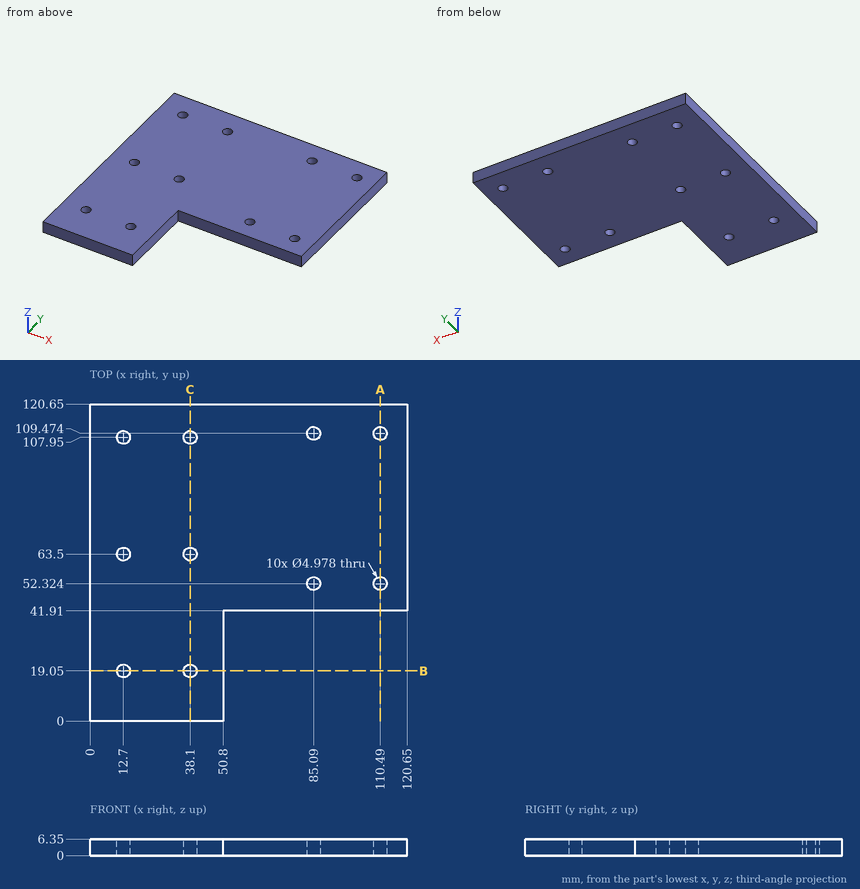
Input: dimensioned drawing with shaded views. Units: mm. Origin: part minimum x, y, z. Give positions to 0.01 mm unless a question says otherwise; leave off trailing zeros. Order: outer loops, then holes, each group sorted by start corner. A loop starts at its lowest first (then second) coordinate and runs counter-clockwise, first axis right, second up. Notation, with made-up numbers: (63, 17.25) -> (72, 17.25) arc R20 ccw to (72, 47.25) -> close; hole circle Ø11 at (61, 54). An arc over 180 degrees is marked (long way). Use a Markdown table: item, result.
1) Section query B-B, the plane y = 19.05. Return the cut outline in (x, z).
Answer list:
| item | result |
|---|---|
| outline | (0, 0) -> (10.21, 0) -> (10.21, 6.35) -> (0, 6.35) -> close; (15.19, 0) -> (35.61, 0) -> (35.61, 6.35) -> (15.19, 6.35) -> close; (40.59, 0) -> (50.8, 0) -> (50.8, 6.35) -> (40.59, 6.35) -> close |
2) Section query C-C, the plane x = 38.1. Return the cut outline in (y, z).
Answer list:
| item | result |
|---|---|
| outline | (0, 0) -> (16.56, 0) -> (16.56, 6.35) -> (0, 6.35) -> close; (21.54, 0) -> (61.01, 0) -> (61.01, 6.35) -> (21.54, 6.35) -> close; (65.99, 0) -> (105.46, 0) -> (105.46, 6.35) -> (65.99, 6.35) -> close; (110.44, 0) -> (120.65, 0) -> (120.65, 6.35) -> (110.44, 6.35) -> close |
3) Section query A-A, the plane x = 110.49. Count the separate pieces of the cut face and the enclosed holes in it, then the cut area to 3 significant figures.
Answer list:
| item | result |
|---|---|
| separate pieces | 3 |
| enclosed holes | 0 |
| area | 437 mm² |
4) Ray query, line 1 along Y through (x, z) = (12.7, 2.25); line 2 along Y through (x, z) = (59.5, 1.75); line 3 along Y through (x, z) = (40, 2.75). Return the intervals inside material, ascending. Write a range as [from, to].
Answer list:
| item | result |
|---|---|
| line 1 | [0, 16.56], [21.54, 61.01], [65.99, 105.46], [110.44, 120.65] |
| line 2 | [41.91, 120.65] |
| line 3 | [0, 17.44], [20.66, 61.89], [65.11, 106.34], [109.56, 120.65] |
5) Contact query for a flat-ended pin moving along its axis: P1, Ø4.5, axis at x = 110.49, y = 109.474, coming from the +Z side. Output: stop coordinate, or through.
Answer list:
| item | result |
|---|---|
| P1 | through |
